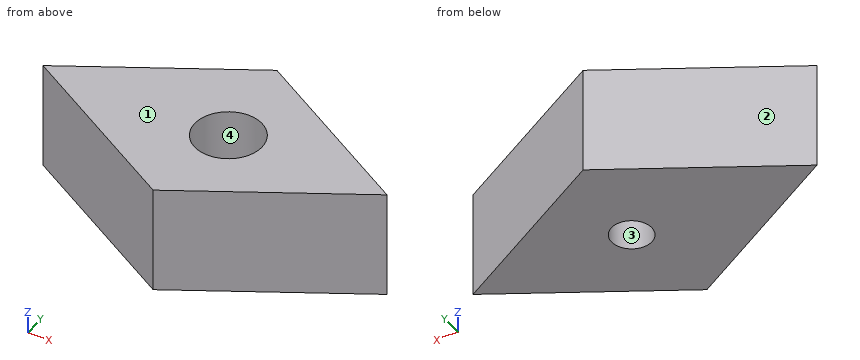
```python
from build123d import *

# Parameters (mm, degrees)
EXTRUDE_1_DEPTH           = 8
HOLE_WIZARD_3_D           = 3
HOLE_WIZARD_3_DEPTH       = 9
HOLE_WIZARD_3_CBORE_D     = 5
HOLE_WIZARD_3_CBORE_DEPTH = 4


with BuildPart() as part:
    # 草图1 → 凸台-拉伸1 (new body)
    with BuildSketch(Plane.XY):
        Polygon((0, 7.5), (-12.990381057, 0), (0, -7.5), (12.990381057, 0), align=None)
    extrude(amount=EXTRUDE_1_DEPTH)

    # 孔3
    with Locations(Plane(origin=(1.009618943, 0, 8), x_dir=(1, 0, 0), z_dir=(0, 0, 1))):
        with Locations((0, 0)):
            CounterBoreHole(HOLE_WIZARD_3_D / 2, HOLE_WIZARD_3_CBORE_D / 2, HOLE_WIZARD_3_CBORE_DEPTH, depth=HOLE_WIZARD_3_DEPTH)


solid = part.part
```
The listing builds one solid part. Answer for the finished solid, in the listing's coordinates (mm). Face numbers are marked on the shaded views. Coordinates: 2 decimals unless noted, no trailing zeros. Write each loop counter-clockwise with the first axis right and the second up, starting at its lowest first coordinate (ties: lowest second). Pieces come first, ordered by that corner, then holes. Notation, with made-up numbers: (31.25, 77.25) - (78.25, 77.25) arc R21 cw to (78.25, 95.25) - close; hole circle Ø10 at (53, 57.25). An arc over 180 degrees is marked (long way). One line per item, written item: value.
1) Find section A-A (z = 3.5). Give the vertices of the cut face in (x, y).
Geometry check:
outline: (-12.99, 0) - (0, -7.5) - (12.99, 0) - (0, 7.5) - close; hole circle Ø3 at (1.01, 0)
2) Find section C-C (z = 6.25). Give the vertices of the cut face in (x, y).
Geometry check:
outline: (-12.99, 0) - (0, -7.5) - (12.99, 0) - (0, 7.5) - close; hole circle Ø5 at (1.01, 0)
3) Find section B-B (y = 3.75). Give the vertices of the cut face in (x, z), and give its area (3 significant figures).
Geometry check:
outline: (-6.5, 0) - (6.5, 0) - (6.5, 8) - (-6.5, 8) - close
area: 104 mm2
4) Consider line 1 along Y through (x, z) = (0.5, 6.75); line 2 along Y through (x, z) = (2, 4.75); line 3 along Y through (x, z) = (4, 7). Determine where each line is inside the solid, lowest interval first. Write a range as from..to.
Geometry check:
line 1: y = -7.21..-2.45, 2.45..7.21
line 2: y = -6.35..-2.3, 2.3..6.35
line 3: y = -5.19..5.19
5) Each of these flat-tipped pins is pushed along its axis until it touches: pin 1 Ø3 at (x, z) = (4, 4.5) entering from +Y; pin 2 Ø1.8 at (x, y) = (1.01, 0) entering from +Z; pin 3 Ø3 at (x, z) = (6.5, 2.5) entering from +Y; pin 4 Ø2 at (y, z) = (-5.5, 3) entering from +X. Where does it stop, or does it pass through?
Geometry check:
pin 1: stops at y = 6.06
pin 2: passes through
pin 3: stops at y = 4.61
pin 4: stops at x = 5.2
6) For a pull along Y with two mould halves and no side action, classify the marked faces 1, 2, 3 and 4 as pulls with the +Y half, pulls with the -Y half, needs draft (parallel to the pull), parting line crosses it, or undercut.
Geometry check:
face 1: needs draft
face 2: pulls with the +Y half
face 3: undercut
face 4: undercut
7) Find section D-D (x = -8.75). Give the vertices of the cut face in (y, z).
Geometry check:
outline: (-2.45, 0) - (2.45, 0) - (2.45, 8) - (-2.45, 8) - close
